Source: CAD feature listing. Evaluate the final solid. Frame: model axes, mm. Give positions to 0.01 mm unless a question says otherwise; leave off trailing zeros. Loops run counter-clockwise (first coordinate to the right, second up) from the corner with the lowest first, then second, coordinate; pieces in that order, holes last. Notation, with made-up numbers: M 74,14 L 114,14 A29 cw 114,41 Z; hole C 37.25,64.25 d9. An arc over 180 degrees is marked long. Answer in a Markdown table with one row per item.
```python
from build123d import *

# Parameters (mm, degrees)
BOSS_EXTRUDE1_DEPTH = 1.6
SKETCH2_W           = 4
SKETCH2_H           = 13
CUT_EXTRUDE2_DEPTH  = 10
SKETCH3_W           = 7.5
SKETCH3_H           = 5.5
CUT_EXTRUDE3_DEPTH  = 10
SKETCH4_R           = 0.75
CUT_EXTRUDE4_DEPTH  = 10


with BuildPart() as part:
    # Sketch1 → Boss-Extrude1 (new body)
    with BuildSketch(Plane(origin=(0, 0, 0), x_dir=(1, 0, 0), z_dir=(0, 1, 0))):
        with BuildLine():
            Line((20, 0), (20, -26))
            Line((20, -26), (-20, -26))
            Line((-20, -26), (-20, 0))
            ThreePointArc((-20, 0), (0, 20), (20, 0))
        make_face()
    extrude(amount=BOSS_EXTRUDE1_DEPTH)

    # Sketch2 → Cut-Extrude2 (cut)
    with BuildSketch(Plane(origin=(0, 3, 0), x_dir=(1, 0, 0), z_dir=(0, 1, 0))):
        with Locations((-18, -9)):
            Rectangle(SKETCH2_W, SKETCH2_H)
        with Locations((18, -9)):
            Rectangle(SKETCH2_W, SKETCH2_H)
    extrude(amount=-CUT_EXTRUDE2_DEPTH, mode=Mode.SUBTRACT)

    # Sketch3 → Cut-Extrude3 (cut)
    with BuildSketch(Plane(origin=(0, 1.6, 0), x_dir=(1, 0, 0), z_dir=(0, 1, 0))):
        with Locations((-9.9, -14.8)):
            Rectangle(SKETCH3_W, SKETCH3_H)
    cut_extrude3 = extrude(amount=-CUT_EXTRUDE3_DEPTH, mode=Mode.SUBTRACT)

    # Mirror1: Cut-Extrude3 across plane
    add(cut_extrude3.mirror(Plane(origin=(0, 0, 0), x_dir=(0, 0, 1), z_dir=(1, 0, 0))), mode=Mode.SUBTRACT)

    # Sketch4 → Cut-Extrude4 (cut)
    with BuildSketch(Plane(origin=(0, 1.6, 0), x_dir=(1, 0, 0), z_dir=(0, 1, 0))):
        with Locations(Location((-14.75, -7, 0), (0, 0, 270))):
            Circle(SKETCH4_R)
        with Locations(Location((-14.75, -11, 0), (0, 0, 270))):
            Circle(SKETCH4_R)
        with Locations(Location((-12.25, -7, 0), (0, 0, 270))):
            Circle(SKETCH4_R)
    cut_extrude4 = extrude(amount=-CUT_EXTRUDE4_DEPTH, mode=Mode.SUBTRACT)

    # Mirror2: Cut-Extrude4 across plane
    add(cut_extrude4.mirror(Plane(origin=(0, 0, 0), x_dir=(0, 0, 1), z_dir=(1, 0, 0))), mode=Mode.SUBTRACT)


solid = part.part
```
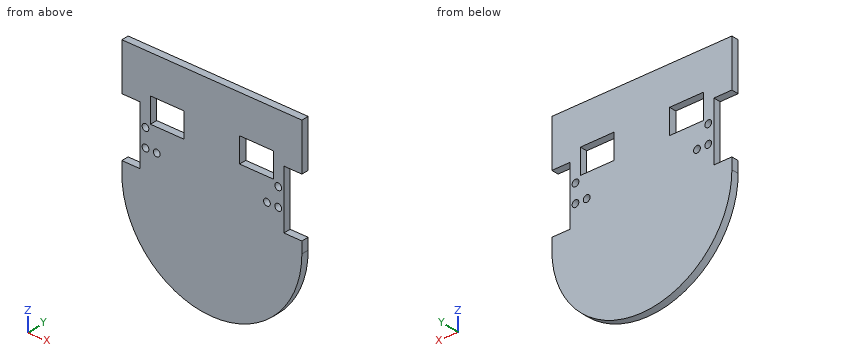
Q1. Section query D-D (x = 14.75). Output: boundary loops of the cut face in (y, z).
Values follow:
| item | result |
|---|---|
| outline | M 0,-13.51 L 1.6,-13.51 L 1.6,6.25 L 0,6.25 Z; M 0,7.75 L 1.6,7.75 L 1.6,10.25 L 0,10.25 Z; M 0,11.75 L 1.6,11.75 L 1.6,26 L 0,26 Z |
Q2. Section query A-A (z = 11). Output: boundary loops of the cut face in (x, y).
Values follow:
| item | result |
|---|---|
| outline | M -16,0 L -15.5,0 L -15.5,1.6 L -16,1.6 Z; M -14,0 L 14,0 L 14,1.6 L -14,1.6 Z; M 15.5,0 L 16,0 L 16,1.6 L 15.5,1.6 Z |
Q3. Ray query, probe 1 along X at (y, z) = (0.8, 7); probe 2 along X at (y, z) = (1.1, 14.5); probe 3 along Z at (x, y) = (14.75, 0.7). Return the intervals inside material, ascending. Write a range as from..to.
Values follow:
| item | result |
|---|---|
| probe 1 | -16..-15.5, -14..-13, -11.5..11.5, 13..14, 15.5..16 |
| probe 2 | -16..-13.65, -6.15..6.15, 13.65..16 |
| probe 3 | -13.51..6.25, 7.75..10.25, 11.75..26 |
Q4. Section query B-B (y = 1.15). Give the number of separate pieces and of enclosed holes in the cut face, plus the area to 3 significant figures.
Values follow:
| item | result |
|---|---|
| separate pieces | 1 |
| enclosed holes | 8 |
| area | 1,470 mm^2 |
Q5. Section query C-C (x = -11). Output: boundary loops of the cut face in (y, z).
Values follow:
| item | result |
|---|---|
| outline | M 0,-16.7 L 1.6,-16.7 L 1.6,12.05 L 0,12.05 Z; M 0,17.55 L 1.6,17.55 L 1.6,26 L 0,26 Z |
Q6. Contact query for flat-ended pins moving along their axis: pin 1 Ø0.9 at (x, z) = (-14.75, 11) entering from +Y (3 decimals); pin 2 Ø0.5 at (y, z) = (0.5, 13.5) entering from +X; pin 3 Ø0.5 at (y, z) = (0.5, 14.5) entering from -X. Output: stop coordinate, or through.
Values follow:
| item | result |
|---|---|
| pin 1 | through |
| pin 2 | x = 16 |
| pin 3 | x = -16 |
